Verification items for the finished model (mm, model axes). A direction names the side the tool comes from. Round coordinates to 2 decimals unless told otherwise and drop trailing zeros. Write each loop counter-clockwise with the first axis right and the second up, starting at its lowest first coordinate (ties: lowest second). Pieces come first, ordered by that corner, then holes. Notation, with made-up numbers: (-12, 88) - (6, 88) arc R31 cw to (6, 116) - close; hole circle Ø10 at (-33.75, 24). An arc over 180 degrees is marked (long way). Answer as a JSON object with one key per item and string values. Group by question number.
1) Set-up check for faces 5 (the flat face through (0, 1, -11)), 6 (the flat face through (-5, 2, -5)): record each of +Z, -Z, +X, -X, +Y, -Y from which the full face is reachable in a straight line by a thin tool's end or side.
2) Section check B-B (y = 1.5). Enter the section's corners in (x, z).
3) Mould release check, pull along X, two halves, no side actions. Record for faces 1 (the cylindrical face through (-6.56, 0.97, 9.66)), 2 (the flat face through (10, 1, 0)), 3 (the flat face through (0, 0, 0)), 4 (the flat face through (-10, 1, 0)): +X half, -X half, draft (parallel to the pull), parting line (faces both ways), or undercut.
4) Section check D-D (z = 3). Enter the section's corners in (x, y).
5) Thickness scan on line 1 (X direction, y = 1.3, z = 8.75); line 2 (Z direction, x = 7.75, y = 1.55); line 3 (Y direction, x = 9, z = 6.25). Record the ranges inside material, lowest first.
6) Go/stop test with flat-tipped pins: pin 1 Ø2.5 at (x, z) = (7.75, 8.75) entering from +Y; pin 2 Ø1.5 at (x, z) = (1.5, -8) entering from +Y; pin 3 Ø1.5 at (x, y) = (-4, 3.5) entering from +Z; pin 4 Ø1 at (y, z) = (10, -4) entering from -X. Record where each tip stops, or that it passes through.
7) Section check C-C (x = 5.5). Enter the section's corners in (y, z), then the cut area to 3 significant figures.
8) Section check A-A (z = -8.75). Enter the section's corners in (x, y) (3 decimals).
```python
from build123d import *

# Parameters (mm, degrees)
SKETCH1_W                          = 20
SKETCH1_H                          = 22
BOSS_EXTRUDE1_DEPTH                = 2
F_3_0_3_DIAMETER_HOLE1_D           = 3
F_3_0_3_DIAMETER_HOLE1_CSINK_D     = 3.05
F_3_0_3_DIAMETER_HOLE1_CSINK_ANGLE = 90
SKETCH4_R                          = 6
BOSS_EXTRUDE2_DEPTH                = 10


with BuildPart() as part:
    # Sketch1 → Boss-Extrude1 (new body)
    with BuildSketch(Plane(origin=(0, 0, 0), x_dir=(1, 0, 0), z_dir=(0, 1, 0))):
        Rectangle(SKETCH1_W, SKETCH1_H)
    extrude(amount=BOSS_EXTRUDE1_DEPTH)

    # Ø3.0 (3) Diameter Hole1 (through all)
    with Locations(Plane(origin=(0, 2, 0), x_dir=(1, 0, 0), z_dir=(0, 1, 0))):
        with Locations((-7.75, 8.75), (7.75, -8.75), (-7.75, -8.75), (7.75, 8.75)):
            CounterSinkHole(F_3_0_3_DIAMETER_HOLE1_D / 2, F_3_0_3_DIAMETER_HOLE1_CSINK_D / 2, counter_sink_angle=F_3_0_3_DIAMETER_HOLE1_CSINK_ANGLE)

    # Sketch4 → Boss-Extrude2 (add)
    with BuildSketch(Plane(origin=(0, 2, 0), x_dir=(1, 0, 0), z_dir=(0, 1, 0))):
        with Locations(Location((0, 0, 0), (0, 0, 270))):
            Circle(SKETCH4_R)
    extrude(amount=BOSS_EXTRUDE2_DEPTH)


solid = part.part
```
Returned:
{
 "1": {"face 5": "-Z, +X, -X, +Y, -Y", "face 6": "+Y"},
 "2": {"outline": "(-10, -11) - (10, -11) - (10, 11) - (-10, 11) - close; hole circle Ø3 at (-7.75, -8.75); hole circle Ø3 at (-7.75, 8.75); hole circle Ø3 at (7.75, -8.75); hole circle Ø3 at (7.75, 8.75)"},
 "3": {"face 1": "undercut", "face 2": "+X half", "face 3": "draft", "face 4": "-X half"},
 "4": {"outline": "(-10, 0) - (10, 0) - (10, 2) - (5.2, 2) - (5.2, 12) - (-5.2, 12) - (-5.2, 2) - (-10, 2) - close"},
 "5": {"line 1": "-10 to -9.25, -6.25 to 6.25, 9.25 to 10", "line 2": "-11 to -10.25, -7.25 to 7.25, 10.25 to 11", "line 3": "0 to 2"},
 "6": {"pin 1": "through", "pin 2": "y = 2", "pin 3": "z = 5.04", "pin 4": "x = -4.87"},
 "7": {"outline": "(0, -11) - (2, -11) - (2, -2.4) - (12, -2.4) - (12, 2.4) - (2, 2.4) - (2, 11) - (0, 11) - close", "area": "92.0 mm2"},
 "8": {"outline": "(-10, 0) - (-9.25, 0) - (-9.25, 1.975) - (-9.275, 2) - (-10, 2) - close; (-6.25, 0) - (6.25, 0) - (6.25, 1.975) - (6.225, 2) - (-6.225, 2) - (-6.25, 1.975) - close; (9.25, 0) - (10, 0) - (10, 2) - (9.275, 2) - (9.25, 1.975) - close"}
}
